```python
from build123d import *

# Parameters (mm, degrees)
F0_W     = 52
F0_H     = 24
F0_R     = 2
F1_DEPTH = 2
F2_W     = 52
F2_H     = 24
F2_W_2   = 48
F2_H_2   = 20
F3_DEPTH = 15
F4_W     = 52
F4_H     = 24
F4_R     = 2
F5_DEPTH = 2
F6_W     = 20
F6_H     = 15
F7_DEPTH = 2


with BuildPart() as f1:
    # F0 (on Top) → F1 (new body)
    with BuildSketch(Plane.XY):
        with Locations((26, 12)):
            Rectangle(F0_W, F0_H)
        with Locations((5, 5)):
            Circle(F0_R, mode=Mode.SUBTRACT)
    extrude(amount=F1_DEPTH)

    # F2 (on face) → F3 (join)
    with BuildSketch(Plane.XY.offset(2)):
        with Locations((26, 12)):
            Rectangle(F2_W, F2_H)
        with Locations((26, 12)):
            Rectangle(F2_W_2, F2_H_2, mode=Mode.SUBTRACT)
    extrude(amount=F3_DEPTH)

    # F4 (on face) → F5 (join)
    with BuildSketch(Plane.XY.offset(17)):
        with Locations((26, 12)):
            Rectangle(F4_W, F4_H)
        with Locations((5, 5)):
            Circle(F4_R, mode=Mode.SUBTRACT)
    extrude(amount=F5_DEPTH)

    # F6 (on face) → F7 (cut, through all)
    with BuildSketch(Plane.YZ.offset(52)):
        with Locations((12, 9.5)):
            Rectangle(F6_W, F6_H)
    extrude(amount=-F7_DEPTH, mode=Mode.SUBTRACT)


solid = f1.part
```
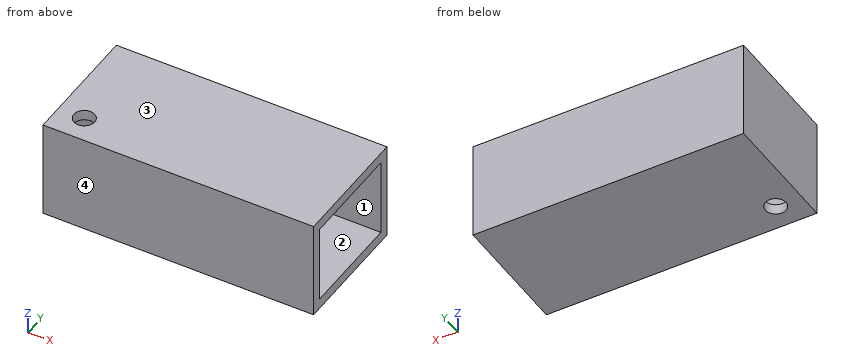
Part model, mm, in its own coordinate system. Face numbers are marked on the shaded views. Round coordinates to 2 decimals unless told otherwise and drop trailing zeros. Order: outer loops, then holes, each group sorted by start corner. A loop starts at its lowest first (then second) coordinate and runs counter-clockwise, first axis right, second up. Notation, with made-up numbers: M 30.25,39 L 77.25,39 A27 cw 77.25,55 Z; hole C -2,68 d10. An arc over 180 degrees is marked long. Answer in a Markdown table with one row per item. Add a question column.
Q1. Cut at C-C on x = 5. Give the cut face in (y, z), and give its area (3 significant figures).
Q2. Cut at D-D on y = 21. Give the cut face in (x, z).
Q3. Mould opens along Z. For the marked faces 1, 2, 3 and 4 say: +Z half, -Z half, draft (parallel to the pull), parting line (faces both ways), or undercut.
Q4. Cut at B-B on y = 5. Give the cut face in (x, z).
Q5. Cut at A-A on x = 45. Give the cut face in (y, z).
Q6. Pin check, flat tips, straight feed: pin 1 (4.5 mm diameter, centred on x = 22, z = 7, fed in from -Y); pin 2 (2.5 mm diameter, centred on x = 5, y = 5, fed in from +Z); pin 3 (1.5 mm diameter, centred on y = 15.5, z = 6.5, fed in from +X). Stop position of each tip, or through.
Q7. Wall check: L1, parallel to Z at x = 33, y = 12.75; L2, parallel to Y at x = 39.5, z = 7.5; L3, parallel to Y at x = 5, z = 17.4. Give the ranges that are in metal, low to high. Write a range as from..to.
Established:
| question | item | result |
|---|---|---|
| 1 | outline | M 0,0 L 3,0 L 3,2 L 2,2 L 2,17 L 3,17 L 3,19 L 0,19 Z; M 7,0 L 24,0 L 24,19 L 7,19 L 7,17 L 22,17 L 22,2 L 7,2 Z |
| 1 | area | 140 mm2 |
| 2 | outline | M 0,0 L 52,0 L 52,2 L 2,2 L 2,17 L 52,17 L 52,19 L 0,19 Z |
| 3 | face 1 | undercut |
| 3 | face 2 | undercut |
| 3 | face 3 | +Z half |
| 3 | face 4 | draft |
| 4 | outline | M 0,0 L 3,0 L 3,2 L 2,2 L 2,17 L 3,17 L 3,19 L 0,19 Z; M 7,0 L 52,0 L 52,2 L 7,2 Z; M 7,17 L 52,17 L 52,19 L 7,19 Z |
| 5 | outline | M 0,0 L 24,0 L 24,19 L 0,19 Z; hole M 2,2 L 22,2 L 22,17 L 2,17 Z |
| 6 | pin 1 | stops at y = 0 |
| 6 | pin 2 | passes through |
| 6 | pin 3 | stops at x = 2 |
| 7 | L1 | z = 0..2, 17..19 |
| 7 | L2 | y = 0..2, 22..24 |
| 7 | L3 | y = 0..3, 7..24 |
